Design review of the part shown in the three views and the two pictorial views. Dimensions are in mm from the part's minimum x, y and z. A direction names the side the tool comes from. Give positions to 0.01 mm unless a question says otherwise; leave off trailing zeros. Loops run counter-clockwise (first coordinate to the right, second up) from the corner with the lowest first, then second, coordinate; pieces in that order, holes last. Notation, with made-up numbers: (59.5, -5.75) - (105.5, -5.75) arc R8 ccw to (105.5, 4.25) - close; hole circle Ø11 at (33.5, 62). An arc over 180 degrees is marked (long way). Answer as a JSON object with one key per item and string values.
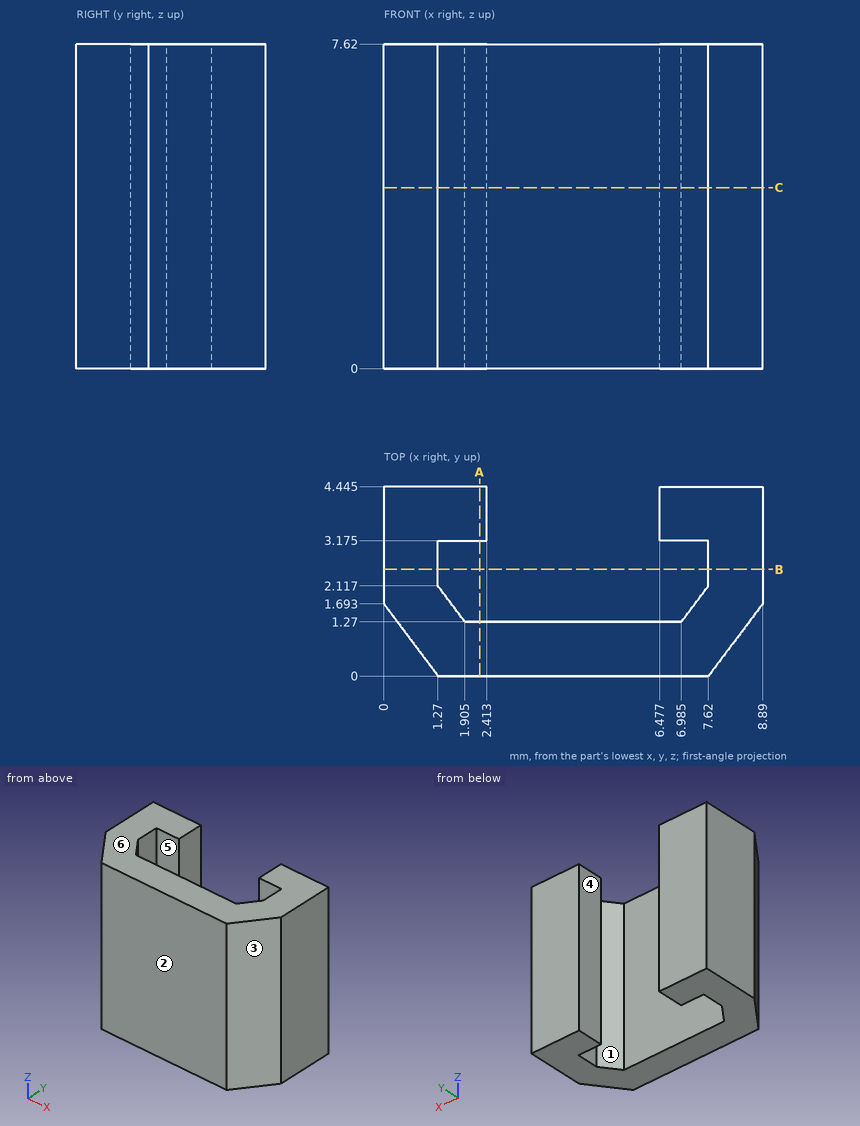
Q1. The part is to be moulded in two halves that separate along X. For the marked faces 1, 2 and 3, say which applies: +X half, -X half, draft (parallel to the pull), parting line (faces both ways), or undercut.
Results:
{"face 1": "undercut", "face 2": "draft", "face 3": "+X half"}
Q2. For the marked faces 4, 5 and 6, list the 3-axis set-ups (+Z, -Z, +X, -X, +Y, -Y) from which the entire face can be reached by the end or side of a thin tool; tool diameter is ignored.
Results:
{"face 4": "+Z, -Z, +Y", "face 5": "+Z, -Z", "face 6": "+Z, +X, -X, +Y, -Y"}
Q3. To check wall thickness, follow probe 1 along X at (y, z) = (2.45, 5.75); probe 2 along X at (y, z) = (3.6, 6); probe 3 along Y at (x, z) = (6.75, 1) (1 decimal). State the ranges of each line that lie inside material, in increasing order. Write a range as [from, to].
Results:
{"probe 1": "x = [0, 1.27], [7.62, 8.89]", "probe 2": "x = [0, 2.41], [6.48, 8.89]", "probe 3": "y = [0, 1.3], [3.2, 4.4]"}
Q4. Consider section C-C, the plane z = 4.25. State the section outline as (x, y) points (1 decimal).
Results:
{"outline": "(0, 1.7) - (1.3, 0) - (7.6, 0) - (8.9, 1.7) - (8.9, 4.4) - (6.5, 4.4) - (6.5, 3.2) - (7.6, 3.2) - (7.6, 2.1) - (7, 1.3) - (1.9, 1.3) - (1.3, 2.1) - (1.3, 3.2) - (2.4, 3.2) - (2.4, 4.4) - (0, 4.4) - close"}
Q5. Consider section B-B, the plane y = 2.5. State the section outline as (x, z) points.
Results:
{"outline": "(0, 0) - (1.27, 0) - (1.27, 7.62) - (0, 7.62) - close; (7.62, 0) - (8.89, 0) - (8.89, 7.62) - (7.62, 7.62) - close"}
Q6. Consider section A-A, the plane x = 2.25. State the section outline as (y, z) points (1 decimal).
Results:
{"outline": "(0, 0) - (1.3, 0) - (1.3, 7.6) - (0, 7.6) - close; (3.2, 0) - (4.4, 0) - (4.4, 7.6) - (3.2, 7.6) - close"}
